Could you check a few things on this drawing? It's one solid part, dimensions in mm from its lowest x, y, z. Coordinates: 2 decimals unless noted, no trailing zeros. Order: outer loops, then holes, each group sorted by start corner. A loop starts at its lowest first (then second) coordinate and runs counter-clockwise, first axis right, second up.
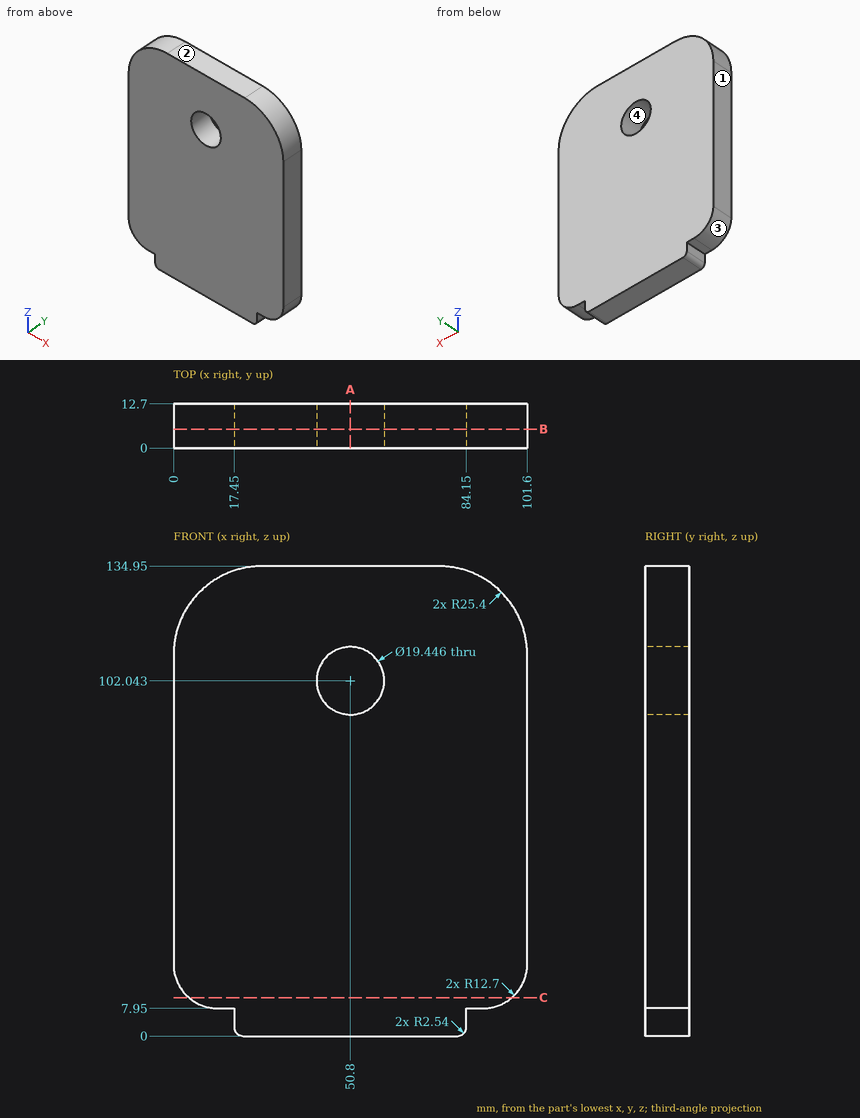
Q1. If we section it at A-A on x = 50.8: Write out the boundary of the cut face in (y, z), then the cut area to 3 significant figures.
Q2. If we section it at B-B on y = 5.5: Write out the boundary of the cut face in (x, z).
Q3. If we section it at C-C on z = 11: Write out the boundary of the cut face in (x, y), then the cut area to 3 significant figures.
Q4. Will these pins go through, and if not, where does the flat tip stop? pin 1 (17.5 mm diameter, centred on x = 50.8, z = 102.04, fed in from -Y); pin 2 (2.5 mm diameter, centred on x = 14, y = 3.5, fed in from -Z).
Q5. I need wall thicknesses on L1, parallel to Z at x = 50.8, y = 6.5; L2, parallel to X at y = 2.5, z = 94 (1 decimal); L3, parallel to Z at x = 46, y = 2. Which ranges of each line are inside material? Lowest first, please.
Q6. We'd pull the mould along Z, two halves only. Please class the marked faces 1, 2, 3 and 4: pulls with the +Z half, pulls with the -Z half, needs draft (parallel to the pull), parting line crosses it, or undercut.
Reply:
1. outline: (0, 0) - (12.7, 0) - (12.7, 92.32) - (0, 92.32) - close; (0, 111.77) - (12.7, 111.77) - (12.7, 134.95) - (0, 134.95) - close
1. area: 1,470 mm2
2. outline: (0, 20.65) arc R12.7 ccw to (12.7, 7.95) - (17.45, 7.95) - (17.45, 2.54) arc R2.54 ccw to (19.99, 0) - (81.61, 0) arc R2.54 ccw to (84.15, 2.54) - (84.15, 7.95) - (88.9, 7.95) arc R12.7 ccw to (101.6, 20.65) - (101.6, 109.55) arc R25.4 ccw to (76.2, 134.95) - (25.4, 134.95) arc R25.4 ccw to (0, 109.55) - close; hole circle Ø19.45 at (50.8, 102.04)
3. outline: (4.44, 0) - (97.16, 0) - (97.16, 12.7) - (4.44, 12.7) - close
3. area: 1,180 mm2
4. pin 1: passes through
4. pin 2: stops at z = 7.95
5. L1: z = 0 to 92.32, 111.77 to 134.95
5. L2: x = 0 to 45.3, 56.3 to 101.6
5. L3: z = 0 to 93.59, 110.5 to 134.95
6. face 1: needs draft
6. face 2: pulls with the +Z half
6. face 3: pulls with the -Z half
6. face 4: undercut
